Model file for the job. Use its own axes, mm. A direction names the side the tool comes from. Round coordinates to 2 decimals unless told otherwise and drop trailing zeros. Order: outer loops, then holes, each group sorted by start corner. A loop starts at its lowest first (then second) coordinate and runs counter-clockwise, first axis right, second up. Notation, with made-up numbers: (-13.75, 79) - (-5.75, 79) arc R30 ccw to (-5.75, 115) - close; hole circle Ø4 at (29, -9.75). An arc over 180 degrees is marked (long way). Answer as CSV lines item,"result". Start each with the question number.
1. Band-saw the part on B-B on y = 9.5. List the corners of the cut face in (x, z), then the cut area to 3 significant figures.
2. Band-saw the part on A-A on z = 0.7. List the corners of the cut face in (x, y), then the cut area to 3 significant figures.
3. Wall check: line 1 along Y through (x, z) = (-15.5, 2.7); line 2 along X through (y, z) = (7, 3.7); line 3 along Y through (x, z) = (-27.5, 2.8). Give the ranges that are in metal, low to high. Write a range as [from, to].
4. 3-axis set-ups, long thin cutter, end or side, ignore diameter. For faces 1 (the face through (2, 32, 3)), 2 (the face through (0.3, 33, 1.5)), 3 (the face through (-25.1, 29.14, 2.99)), 4 (the face through (0, -33, 2)): which of +Z, -Z, +X, -X, +Y, -Y reach the whole face in a straight line?
5. Pull direction X, two halves, no side cores. Call faces 5 (the face through (-29, 0, 2)), 6 (the face through (29, 0, 2)), 7 (the face through (25.14, 29.1, 2.99)): released by +X, released by -X, zero draft, split by the parting line, or undercut.
6. Band-saw the part on C-C on x = 10. List the corners of the cut face in (y, z), then the cut area to 3 significant figures.
7. Pin check, flat tips, straight feed: pin 1 Ø0.6 at (y, z) = (-12, 3.5) entering from -X; pin 2 Ø0.6 at (y, z) = (32, 2.5) entering from -X; pin 3 Ø1 at (y, z) = (31.5, 3.5) entering from +X; pin 4 Ø3.5 at (x, y) = (-29, -33) entering from +Z. Stop position of each tip, or through.
```python
from build123d import *

# Parameters (mm, degrees)
F2_DEPTH = 4
F3_W     = 4
F3_H     = 2
F4_DEPTH = 4
F5_W     = 52
F5_H     = 60
F6_DEPTH = 2
F7_R     = 2
F8_DEPTH = 4
F9_R     = 3


with BuildPart() as f2:
    # F1 (on Top) → F2 (new body)
    with BuildSketch(Plane.XY):
        with BuildLine():
            ThreePointArc((-29, 29), (-26.1715728753, 30.1715728753), (-25, 33))
            Line((-25, 33), (-29, 33))
            Line((-29, 33), (-29, 29))
        make_face()
        with BuildLine():
            Line((-29, 33), (-25, 33))
            ThreePointArc((-25, 33), (-31.8284271247, 35.8284271247), (-29, 29))
            Line((-29, 29), (-29, 33))
        make_face()
        with BuildLine():
            Line((25, 33), (-25, 33))
            ThreePointArc((-25, 33), (-26.1715728753, 30.1715728753), (-29, 29))
            Line((-29, 29), (-29, -29))
            ThreePointArc((-29, -29), (-26.1715728753, -30.1715728753), (-25, -33))
            Line((-25, -33), (25, -33))
            ThreePointArc((25, -33), (26.1715728753, -30.1715728753), (29, -29))
            Line((29, -29), (29, 29))
            ThreePointArc((29, 29), (26.1715728753, 30.1715728753), (25, 33))
        make_face()
        with BuildLine():
            ThreePointArc((33, 33), (29, 37), (25, 33))
            Line((25, 33), (29, 33))
            Line((29, 33), (29, 29))
            ThreePointArc((29, 29), (31.8284271247, 30.1715728753), (33, 33))
        make_face()
        with BuildLine():
            Line((29, 33), (25, 33))
            ThreePointArc((25, 33), (26.1715728753, 30.1715728753), (29, 29))
            Line((29, 29), (29, 33))
        make_face()
        with BuildLine():
            ThreePointArc((-25, -33), (-26.1715728753, -30.1715728753), (-29, -29))
            Line((-29, -29), (-29, -33))
            Line((-29, -33), (-25, -33))
        make_face()
        with BuildLine():
            Line((-29, -33), (-29, -29))
            ThreePointArc((-29, -29), (-31.8284271247, -35.8284271247), (-25, -33))
            Line((-25, -33), (-29, -33))
        make_face()
        with BuildLine():
            ThreePointArc((33, -33), (31.8284271247, -30.1715728753), (29, -29))
            Line((29, -29), (29, -33))
            Line((29, -33), (25, -33))
            ThreePointArc((25, -33), (29, -37), (33, -33))
        make_face()
        with BuildLine():
            Line((29, -33), (29, -29))
            ThreePointArc((29, -29), (26.1715728753, -30.1715728753), (25, -33))
            Line((25, -33), (29, -33))
        make_face()
    extrude(amount=F2_DEPTH)

    # F3 (on face) → F4 (cut)
    with BuildSketch(Plane(origin=(0, 33, 0), x_dir=(-1, 0, 0), z_dir=(0, 1, 0))):
        with Locations((0, 3)):
            Rectangle(F3_W, F3_H)
    extrude(amount=-F4_DEPTH, mode=Mode.SUBTRACT)

    # F5 (on face) → F6 (cut)
    with BuildSketch(Plane.XY.offset(4)):
        Rectangle(F5_W, F5_H)
    extrude(amount=-F6_DEPTH, mode=Mode.SUBTRACT)

    # F7 (on Top) → F8 (cut)
    with BuildSketch(Plane.XY):
        with Locations((29, 33)):
            Circle(F7_R)
        with Locations((-29, 33)):
            Circle(F7_R)
        with Locations((29, -33)):
            Circle(F7_R)
        with Locations((-29, -33)):
            Circle(F7_R)
    extrude(amount=F8_DEPTH, mode=Mode.SUBTRACT)

    # F9
    f9_edges = [f2.edges().sort_by_distance(p)[0] for p in [
        (26, -30, 3),
        (-26, -30, 3),
        (-26, 30, 3),
        (26, 30, 3),
    ]]
    fillet(f9_edges, radius=F9_R)


solid = f2.part
```
Reply:
1,outline,"(-29, 0) - (29, 0) - (29, 4) - (26, 4) - (26, 2) - (-26, 2) - (-26, 4) - (-29, 4) - close"
1,area,"128 mm2"
2,outline,"(-29, -29) arc R4 ccw (long way) to (-25, -33) - (25, -33) arc R4 ccw (long way) to (29, -29) - (29, 29) arc R4 ccw (long way) to (25, 33) - (-25, 33) arc R4 ccw (long way) to (-29, 29) - close; hole circle Ø4 at (-29, -33); hole circle Ø4 at (-29, 33); hole circle Ø4 at (29, -33); hole circle Ø4 at (29, 33)"
2,area,"3,930 mm2"
3,line 1,"y = [-33, -30], [30, 33]"
3,line 2,"x = [-29, -26], [26, 29]"
3,line 3,"y = [-36.71, -34.32], [-31.68, 31.68], [34.32, 36.71]"
4,face 1,"+Z, +Y"
4,face 2,"+Z, -Z, +Y"
4,face 3,"+Z"
4,face 4,"+Z, -Z, -Y"
5,face 5,"released by -X"
5,face 6,"released by +X"
5,face 7,"undercut"
6,outline,"(-33, 0) - (33, 0) - (33, 4) - (30, 4) - (30, 2) - (-30, 2) - (-30, 4) - (-33, 4) - close"
6,area,"144 mm2"
7,pin 1,"stops at x = -29"
7,pin 2,"stops at x = -32.94"
7,pin 3,"stops at x = 32.87"
7,pin 4,"passes through"
